Verification items for the finished model (mm, model axes). Face numbers are marked on the shaded views. A direction names the side the tool comes from. Give positions to 0.01 mm unless a question says otherwise; leave off trailing zeros. Write each loop counter-clockwise with the first axis right and the second up, starting at its lowest first coordinate (ties: lowest second). Pieces come first, ordered by that corner, then holes. Notation, with made-up numbers: (13.5, 24.25) -> (71.5, 24.25) arc R14 ccw to (71.5, 48.25) -> close; hole circle Ø2 at (66.5, -19.5). An arc over 180 degrees is marked (long way). Write item = value, one per line.
from build123d import *
from build123d.topology import SkipClean

# Parameters (mm, degrees)
BOSS_EXTRUDE1_DEPTH     = 8.55
SKETCH2_W               = 10.7
SKETCH2_H               = 10.8
CUT_EXTRUDE1_DEPTH      = 17
SKETCH3_R               = 6
BOSS_EXTRUDE2_DEPTH     = 18
SKETCH4_R               = 4.2
CUT_EXTRUDE2_DEPTH      = 25.239275979
BOSS_EXTRUDE5_DEPTH     = 17.1
SKETCH7_R               = 2.2
CUT_EXTRUDE3_DEPTH      = 40.626944786
CUT_EXTRUDE4_REACH      = 33.94
SKETCH10_W              = 8.106
SKETCH10_H              = 1.5
SKETCH11_W              = 6.997
SKETCH11_H              = 1
CUT_EXTRUDE5_DEPTH      = 27.591587091
CUT_EXTRUDE6_REACH      = 42.967
CUT_EXTRUDE6_END_RADIUS = 6
CUT_EXTRUDE7_START      = -16.8
CUT_EXTRUDE7_DEPTH      = 16.8
BOSS_EXTRUDE6_DEPTH     = 1.553
BOSS_EXTRUDE7_REACH     = 36.128
CUT_EXTRUDE8_START      = -16.8
CUT_EXTRUDE8_DEPTH      = 16.8
CUT_EXTRUDE9_REACH      = 43.851


with BuildPart() as part:
    # Sketch1 → Boss-Extrude1 (new, symmetric)
    with BuildSketch(Plane(origin=(0, 0, 0), x_dir=(0, 0, -1), z_dir=(1, 0, 0))):
        Polygon((0, 0), (0, -3), (-16.0587, -13.8), (-35, -13.8), (-35, 0), align=None)
    extrude(amount=BOSS_EXTRUDE1_DEPTH, both=True)

    # Sketch2 → Cut-Extrude1 (cut)
    with BuildSketch(Plane.XY.offset(35)):
        with Locations((0, -5.4)):
            Rectangle(SKETCH2_W, SKETCH2_H)
    extrude(amount=-CUT_EXTRUDE1_DEPTH, mode=Mode.SUBTRACT)

    # Sketch3 → Boss-Extrude2 (add, through all)
    with BuildSketch(Plane.XY.offset(18)):
        with Locations((0, -0.30175)):
            Circle(SKETCH3_R)
    extrude(amount=-BOSS_EXTRUDE2_DEPTH)

    # Sketch4 → Cut-Extrude2 (cut, through all)
    with BuildSketch(Plane.XY.offset(18)):
        with Locations((0, -0.30175)):
            Circle(SKETCH4_R)
    extrude(amount=-CUT_EXTRUDE2_DEPTH, mode=Mode.SUBTRACT)

    # Sketch8 → Boss-Extrude5 (add, through all)
    with BuildSketch(Plane(origin=(8.55, 0, 0), x_dir=(0, 0, -1), z_dir=(1, 0, 0))):
        Polygon((-26.702, -13.8), (-26.702, -15.3), (-25.702, -15.3), (-24.202, -13.8), align=None)
        Polygon((-16.0587, -13.8), (-15.002, -13.8), (-15.002, -14.8), (-14.002, -14.8), (-13, -13.8), (-11.045997115, -10.428793666), align=None)
    extrude(amount=-BOSS_EXTRUDE5_DEPTH)

    # Sketch7 → Cut-Extrude3 (cut, through all)
    with BuildSketch(Plane(origin=(0, -10.8, 0), x_dir=(1, 0, 0), z_dir=(0, 1, 0))):
        with Locations(Location((0, -25, 0), (0, 0, 180))):
            Circle(SKETCH7_R)
    extrude(amount=-CUT_EXTRUDE3_DEPTH, mode=Mode.SUBTRACT)

    # Cut-Extrude4: up to this plane
    cut_extrude4_end = Plane(origin=(-8.55, -15.3, 25.702), z_dir=(0, -0.7071067811865471, -0.707106781186548))
    # Sketch10 → Cut-Extrude4 (cut, up to the surface)
    with BuildSketch(Plane.XY.offset(26.702), mode=Mode.PRIVATE) as cut_extrude4_sk1:
        with Locations((0, -14.55)):
            Rectangle(SKETCH10_W, SKETCH10_H)
    cut_extrude4_tool1 = split(extrude(cut_extrude4_sk1.sketch, amount=-CUT_EXTRUDE4_REACH, mode=Mode.PRIVATE), bisect_by=cut_extrude4_end, keep=Keep.BOTH, mode=Mode.PRIVATE)
    add(cut_extrude4_tool1.solids().sort_by_distance((0, -14.55, 26.702))[0], mode=Mode.SUBTRACT)

    # Sketch11 → Cut-Extrude5 (cut, through all)
    with BuildSketch(Plane.XY.offset(15.002)):
        with Locations((-5.0515, -14.3)):
            Rectangle(SKETCH11_W, SKETCH11_H)
        with Locations((5.0515, -14.3)):
            Rectangle(SKETCH11_W, SKETCH11_H)
    extrude(amount=-CUT_EXTRUDE5_DEPTH, mode=Mode.SUBTRACT)

    # Cut-Extrude6: up to this cylinder (the profile starts outside it)
    cut_extrude6_end = Plane(origin=(0, -0.30175, 7.230062), z_dir=(0, 0, 1)) * Cylinder(CUT_EXTRUDE6_END_RADIUS, 98.934, mode=Mode.PRIVATE)
    # Sketch12 → Cut-Extrude6 (cut, up to the surface)
    with BuildSketch(Plane.XZ.offset(13.8), mode=Mode.PRIVATE) as cut_extrude6_sk1:
        Polygon((-1.553, 13), (-5.353, 16.8), (-5.353, 0), (5.353, 0), (5.353, 16.8), (1.553, 13), align=None)
    cut_extrude6_tool1 = extrude(cut_extrude6_sk1.sketch, amount=-CUT_EXTRUDE6_REACH, mode=Mode.PRIVATE) - cut_extrude6_end
    add(cut_extrude6_tool1.solids().sort_by_distance((0, -13.8, 7.230062))[0], mode=Mode.SUBTRACT)

    # Sketch13 → Cut-Extrude7 (cut)
    with SkipClean():  # the faces are left unmerged after this step: merging them gives an invalid solid
        with BuildSketch(Plane(origin=(0, 0, 0), x_dir=(-1, 0, 0), z_dir=(0, 0, -1)).offset(CUT_EXTRUDE7_START)):
            with BuildLine():
                Line((-5.359052802, -3), (-5.353, -10.428793666))
                Line((-5.353, -10.428793666), (5.353, -10.428793666))
                Line((5.353, -10.428793666), (5.359052802, -3))
                ThreePointArc((5.359052802, -3), (0, -6.30175), (-5.359052802, -3))
            make_face()
        extrude(amount=CUT_EXTRUDE7_DEPTH, mode=Mode.SUBTRACT)

    # Sketch14 → Boss-Extrude6 (add, symmetric)
    with SkipClean():  # the faces are left unmerged after this step: merging them gives an invalid solid
        with BuildSketch(Plane(origin=(0, 0, 0), x_dir=(0, 0, -1), z_dir=(1, 0, 0))):
            Polygon((-13, -13.8), (-8.073269662, -5.3), (-16.8, -5.3), (-16.8, -13.8), align=None)
        extrude(amount=BOSS_EXTRUDE6_DEPTH, both=True)

    # Sketch15 → Boss-Extrude7 (add, up to next)
    with BuildSketch(Plane(origin=(-7.436377386, -6.523873454, 7.436377386), x_dir=(-0.7993387140757535, 0.3962687040508023, -0.4516953999872244), z_dir=(0.6008807037838052, 0.5271477588310114, -0.6008807037838052)), mode=Mode.PRIVATE) as boss_extrude7_sk1:
        Polygon((-11.246017774, 0.733681451), (-11.246017774, 6.495798547), (-15.999947407, 3.239704803), align=None)
    boss_extrude7_tool1 = extrude(boss_extrude7_sk1.sketch, amount=-BOSS_EXTRUDE7_REACH, mode=Mode.PRIVATE) - part.part
    boss_extrude7 = boss_extrude7_tool1.solids().sort_by_distance((2.819667, -8.984956, 15.533333))[0]
    add(boss_extrude7)

    # Mirror1: Boss-Extrude7 across plane
    with SkipClean():  # the faces are left unmerged after this step: merging them gives an invalid solid
        add(boss_extrude7.mirror(Plane(origin=(0, 0, 0), x_dir=(0, 0, 1), z_dir=(1, 0, 0))))

    # Sketch16 → Cut-Extrude8 (cut)
    with SkipClean():  # the faces are left unmerged after this step: merging them gives an invalid solid
        with BuildSketch(Plane(origin=(0, 0, 0), x_dir=(-1, 0, 0), z_dir=(0, 0, -1)).offset(CUT_EXTRUDE8_START)):
            with BuildLine():
                Line((5.992407441, 0), (8.55, 0))
                Line((8.55, 0), (8.55, -13.8))
                Line((8.55, -13.8), (5.353, -13.8))
                Line((5.353, -13.8), (5.353, -3.011988181))
                ThreePointArc((5.353, -3.011988181), (5.869206565, -1.547709188), (5.992407441, 0))
            make_face()
        extrude(amount=CUT_EXTRUDE8_DEPTH, mode=Mode.SUBTRACT)

    # Sketch17 → Cut-Extrude9 (cut, up to next)
    with BuildSketch(Plane(origin=(8.55, 0, 0), x_dir=(0, 0, -1), z_dir=(1, 0, 0)), mode=Mode.PRIVATE) as cut_extrude9_sk1:
        Polygon((-11.045997115, -10.428793666), (-13, -13.8), (-16.0587, -13.8), align=None)
    cut_extrude9_tool1 = extrude(cut_extrude9_sk1.sketch, amount=-CUT_EXTRUDE9_REACH, mode=Mode.PRIVATE) & part.part
    add(cut_extrude9_tool1.solids().sort_by_distance((8.55, -12.676265, 13.368232))[0], mode=Mode.SUBTRACT)


solid = part.part
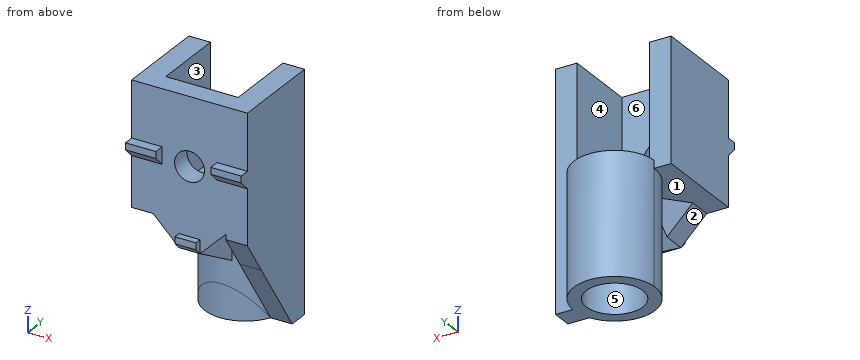
Item 1: Set-up check for the marked faces 1, 2 and 3: record each of +Z, -Z, +X, -X, +Y, -Y from which the full face is reachable in a straight line by a thin tool's end or side.
Response values:
face_1 = -Z, -X
face_2 = -Z, -X, -Y
face_3 = +Z, +Y
Item 2: Sectioned sample at B-B on x = 0. Record the cut outline in (y, z), then the cut area to 3 significant figures.
Response values:
outline = (-14.8, 14) -> (-13.8, 13) -> (-6.3, 8.65) -> (-6.3, 0) -> (-4.5, 0) -> (-4.5, 18) -> (-10.8, 18) -> (-10.8, 22.8) -> (-13.8, 22.8) -> (-13.8, 15) -> (-14.8, 15) -> close; (-13.8, 27.2) -> (-10.8, 27.2) -> (-10.8, 35) -> (-13.8, 35) -> close; (3.9, 0) -> (5.7, 0) -> (5.7, 18) -> (3.9, 18) -> close
area = 158 mm^2
Item 3: Sectioned sample at A-A on z = 25. Record the cut outline in (x, y), then the cut area to 3 significant figures.
Response values:
outline = (-8.55, -14.6) -> (-4.05, -14.6) -> (-4.05, -13.8) -> (-2.2, -13.8) -> (-2.2, -10.8) -> (-5.35, -10.8) -> (-5.35, 0) -> (-8.55, 0) -> close; (2.2, -13.8) -> (4.05, -13.8) -> (4.05, -14.6) -> (8.55, -14.6) -> (8.55, 0) -> (5.35, 0) -> (5.35, -10.8) -> (2.2, -10.8) -> close
area = 114 mm^2
Item 4: Mould release check, pull along Y, two halves, no side actions. Record for the marked faces 4, 5 and 6: +Y half, -Y half, draft (parallel to the pull), parting line (faces both ways), or undercut.
Response values:
face_4 = draft
face_5 = undercut
face_6 = +Y half
Item 5: Sectioned sample at D-D on y = -3.5. Record the cut outline in (x, z).
Response values:
outline = (-8.55, 16.8) -> (-5.08, 16.8) -> (-5.08, 0) -> (-2.72, 0) -> (-2.72, 18) -> (-5.35, 18) -> (-5.35, 35) -> (-8.55, 35) -> close; (2.72, 0) -> (5.08, 0) -> (5.08, 16.8) -> (5.36, 16.8) -> (5.36, 0.74) -> (8.55, 0.74) -> (8.55, 35) -> (5.35, 35) -> (5.35, 18) -> (2.72, 18) -> close
Item 6: Sectioned sample at C-C on z = 30. Record the cut outline in (x, y).
Response values:
outline = (-8.55, -13.8) -> (8.55, -13.8) -> (8.55, 0) -> (5.35, 0) -> (5.35, -10.8) -> (-5.35, -10.8) -> (-5.35, 0) -> (-8.55, 0) -> close
Item 7: Material ranges on line 1 (X direction, y = -4.75, z = 22); line 2 (Y direction, x = 0, z = 14.25); line 3 (Y direction, x = 5.5, z = 28), recorded low to high.
Response values:
line_1 = -8.55 to -5.35, 5.35 to 8.55
line_2 = -14.8 to -4.5, 3.9 to 5.7
line_3 = -13.8 to 0
Item 8: Go/stop test with flat-tipped pins: P1, Ø4, axis at y = -10, z = 13, coming from the -X side; P2, Ø2.5, axis at x = 0, z = 25, coming from the +Y side; P3, Ø2, axis at x = -6.5, y = -3.5, coming from the -Z side; P4, Ø1.5, axis at x = -3.5, z = 29, coming from the +Y side. Record where each tip stops, or that it passes through.
Response values:
P1 = -3.51
P2 = through
P3 = 16.8
P4 = -10.8
